For this review, take the finished solid that the model builds, in its own axes (mm). Face numbers are marked on the shaded views. A direction names the side the tool comes from. Coordinates: 2 decimals unless noted, no trailing zeros. Loops run counter-clockwise (first coordinate to the right, second up) from the corner with the lowest first, then second, coordinate; pieces in that order, holes last. Notation, with made-up numbers: M 19.25,-28.75 L 39.25,-28.75 A20 ccw 39.25,-23.75 Z; hole C 49,-29 d10. An arc over 180 degrees is marked long. Use one line per item in the form item = value.
```python
from build123d import *

# Parameters (mm, degrees)
SKETCH1_R                = 17.5
SKETCH1_R_2              = 1.45
FRONTPANEL_DEPTH         = 4
SKETCH1_3_R              = 34.7
SIDEWALLS_DEPTH          = 28.5
SKETCH2_R                = 19
MOTORSPACER_DEPTH        = 2
SKETCH1_5_R              = 1.45
MOTORMOUNTINGHOLES_DEPTH = 6
BOSS_EXTRUDE7_START      = -6.8
BOSS_EXTRUDE7_DEPTH      = 6.8
SKETCH3_5_R              = 2.2
CUT_EXTRUDE2_DEPTH       = 6
CUT_EXTRUDE8_DEPTH       = 65.705100263
SKETCH11_W               = 34
SKETCH11_H               = 28.5
BOSS_EXTRUDE8_DEPTH      = 10
SKETCH14_W               = 34
SKETCH14_H               = 31.5
BOSS_EXTRUDE9_DEPTH      = 1
CUT_EXTRUDE11_DEPTH      = 1
CUT_EXTRUDE11_DEPTH_BACK = 16
SKETCH19_R               = 10
SKETCH19_R_2             = 6
BOSS_EXTRUDE10_DEPTH     = 50
CUT_EXTRUDE12_REACH      = 227.811
CUT_EXTRUDE14_START      = -5
CUT_EXTRUDE14_DEPTH      = 215.755546028
CUT_EXTRUDE15_START      = -10
SKETCH19_6_R             = 6
CUT_EXTRUDE15_DEPTH      = 30


with BuildPart() as part:
    # Sketch1 → FrontPanel (new body)
    with BuildSketch(Plane.XY):
        with BuildLine():
            Line((-17, 34.543450899), (-17, 43.5))
            Line((-17, 43.5), (17, 43.5))
            Line((17, 43.5), (17, 34.543450899))
            ThreePointArc((17, 34.543450899), (0, -38.5), (-17, 34.543450899))
        make_face()
        Circle(SKETCH1_R, mode=Mode.SUBTRACT)
        with Locations((-7.749339505, 18.708560533)):
            Circle(SKETCH1_R_2, mode=Mode.SUBTRACT)
        with Locations((7.749339505, 18.708560533)):
            Circle(SKETCH1_R_2, mode=Mode.SUBTRACT)
        with Locations((18.708560533, 7.749339505)):
            Circle(SKETCH1_R_2, mode=Mode.SUBTRACT)
        with Locations((18.708560533, -7.749339505)):
            Circle(SKETCH1_R_2, mode=Mode.SUBTRACT)
        with Locations((7.749339505, -18.708560533)):
            Circle(SKETCH1_R_2, mode=Mode.SUBTRACT)
        with Locations((-7.749339505, -18.708560533)):
            Circle(SKETCH1_R_2, mode=Mode.SUBTRACT)
        with Locations((-18.708560533, -7.749339505)):
            Circle(SKETCH1_R_2, mode=Mode.SUBTRACT)
        with Locations((-18.708560533, 7.749339505)):
            Circle(SKETCH1_R_2, mode=Mode.SUBTRACT)
    extrude(amount=FRONTPANEL_DEPTH)

    # Sketch1<3> → SideWalls (add)
    with BuildSketch(Plane.XY):
        with BuildLine():
            Line((-17, 34.543450899), (-17, 43.5))
            Line((-17, 43.5), (17, 43.5))
            Line((17, 43.5), (17, 34.543450899))
            ThreePointArc((17, 34.543450899), (0, -38.5), (-17, 34.543450899))
        make_face()
        with Locations(Location((0, 0, 0), (0, 0, 180))):
            Circle(SKETCH1_3_R, mode=Mode.SUBTRACT)
    extrude(amount=SIDEWALLS_DEPTH)

    # Sketch2 → MotorSpacer (add)
    with BuildSketch(Plane.XY.offset(4)):
        with BuildLine():
            ThreePointArc((-5.4209, 21.321675431), (-9.088731519, 21.942138897), (-11.243546134, 18.909856434))
            ThreePointArc((-11.243546134, 18.909856434), (-15.556349186, 15.556349186), (-18.909856434, 11.243546134))
            ThreePointArc((-18.909856434, 11.243546134), (-21.942138897, 9.088731519), (-21.321675431, 5.4209))
            ThreePointArc((-21.321675431, 5.4209), (-22, 0), (-21.321675431, -5.4209))
            ThreePointArc((-21.321675431, -5.4209), (-21.942138897, -9.088731519), (-18.909856434, -11.243546134))
            ThreePointArc((-18.909856434, -11.243546134), (-15.556349186, -15.556349186), (-11.243546134, -18.909856434))
            ThreePointArc((-11.243546134, -18.909856434), (-9.088731519, -21.942138897), (-5.4209, -21.321675431))
            ThreePointArc((-5.4209, -21.321675431), (0, -22), (5.4209, -21.321675431))
            ThreePointArc((5.4209, -21.321675431), (9.088731519, -21.942138897), (11.243546134, -18.909856434))
            ThreePointArc((11.243546134, -18.909856434), (15.556349186, -15.556349186), (18.909856434, -11.243546134))
            ThreePointArc((18.909856434, -11.243546134), (21.942138897, -9.088731519), (21.321675431, -5.4209))
            ThreePointArc((21.321675431, -5.4209), (22, 0), (21.321675431, 5.4209))
            ThreePointArc((21.321675431, 5.4209), (21.942138897, 9.088731519), (18.909856434, 11.243546134))
            ThreePointArc((18.909856434, 11.243546134), (15.556349186, 15.556349186), (11.243546134, 18.909856434))
            ThreePointArc((11.243546134, 18.909856434), (9.088731519, 21.942138897), (5.4209, 21.321675431))
            ThreePointArc((5.4209, 21.321675431), (0, 22), (-5.4209, 21.321675431))
        make_face()
        with Locations(Location((0, 0, 0), (0, 0, 159.646622112))):
            Circle(SKETCH2_R, mode=Mode.SUBTRACT)
    extrude(amount=MOTORSPACER_DEPTH)

    # Sketch1<5> → MotorMountingHoles (cut)
    with BuildSketch(Plane.XY):
        with Locations(Location((-7.749339505, 18.708560533, 0), (0, 0, 263.105901259))):
            Circle(SKETCH1_5_R)
        with Locations(Location((7.749339505, 18.708560533, 0), (0, 0, 218.105901259))):
            Circle(SKETCH1_5_R)
        with Locations(Location((18.708560533, 7.749339505, 0), (0, 0, 173.105901259))):
            Circle(SKETCH1_5_R)
        with Locations(Location((18.708560533, -7.749339505, 0), (0, 0, 186.894098741))):
            Circle(SKETCH1_5_R)
        with Locations(Location((7.749339505, -18.708560533, 0), (0, 0, 141.894098741))):
            Circle(SKETCH1_5_R)
        with Locations(Location((-7.749339505, -18.708560533, 0), (0, 0, 96.894098741))):
            Circle(SKETCH1_5_R)
        with Locations(Location((-18.708560533, -7.749339505, 0), (0, 0, 51.894098741))):
            Circle(SKETCH1_5_R)
        with Locations(Location((-18.708560533, 7.749339505, 0), (0, 0, 308.105901259))):
            Circle(SKETCH1_5_R)
    extrude(amount=MOTORMOUNTINGHOLES_DEPTH, mode=Mode.SUBTRACT)

    # Sketch3 → Boss-Extrude7 (add)
    with BuildSketch(Plane.XY.offset(28.5).offset(BOSS_EXTRUDE7_START)):
        with BuildLine():
            Line((-21.775846711, 31.75), (-34.3, 31.75))
            Line((-34.3, 31.75), (-34.3, 17.485994396))
            ThreePointArc((-34.3, 17.485994396), (-28.930790001, 25.401956419), (-21.775846711, 31.75))
        make_face()
        with BuildLine():
            Line((34.3, 17.485994396), (34.3, 31.75))
            Line((34.3, 31.75), (21.775846711, 31.75))
            ThreePointArc((21.775846711, 31.75), (28.930790001, 25.401956419), (34.3, 17.485994396))
        make_face()
        with BuildLine():
            Line((-34.3, -17.485994396), (-34.3, -31.75))
            Line((-34.3, -31.75), (-21.775846711, -31.75))
            ThreePointArc((-21.775846711, -31.75), (-28.930790001, -25.401956419), (-34.3, -17.485994396))
        make_face()
        with BuildLine():
            Line((21.775846711, -31.75), (34.3, -31.75))
            Line((34.3, -31.75), (34.3, -17.485994396))
            ThreePointArc((34.3, -17.485994396), (28.930790001, -25.401956419), (21.775846711, -31.75))
        make_face()
    extrude(amount=BOSS_EXTRUDE7_DEPTH)

    # Sketch3<5> → Cut-Extrude2 (cut)
    with BuildSketch(Plane.XY.offset(28.5)):
        with Locations((-28.3, 25.75)):
            Circle(SKETCH3_5_R)
        with Locations(Location((28.3, 25.75, 0), (0, 0, 180))):
            Circle(SKETCH3_5_R)
        with Locations(Location((-28.3, -25.75, 0), (0, 0, 180))):
            Circle(SKETCH3_5_R)
        with Locations((28.3, -25.75)):
            Circle(SKETCH3_5_R)
    extrude(amount=-CUT_EXTRUDE2_DEPTH, mode=Mode.SUBTRACT)

    # Sketch7 → Cut-Extrude8 (cut, through all)
    with BuildSketch(Plane.XY.offset(28.5)):
        with BuildLine():
            Line((-4, 39.7), (4, 39.7))
            ThreePointArc((4, 39.7), (5.5, 38.2), (4, 36.7))
            Line((4, 36.7), (-4, 36.7))
            ThreePointArc((-4, 36.7), (-5.5, 38.2), (-4, 39.7))
        make_face()
    extrude(amount=-CUT_EXTRUDE8_DEPTH, mode=Mode.SUBTRACT)

    # Sketch14 → Boss-Extrude9 (add)
    with BuildSketch(Plane(origin=(0, 43.5, 0), x_dir=(1, 0, 0), z_dir=(0, 1, 0))):
        with Locations((0, -15.75)):
            Rectangle(SKETCH14_W, SKETCH14_H)
    extrude(amount=BOSS_EXTRUDE9_DEPTH)



with BuildPart() as body_2:
    # Sketch11 → Boss-Extrude8 (new body)
    with BuildSketch(Plane(origin=(0, 65, 0), x_dir=(1, 0, 0), z_dir=(0, 1, 0))):
        with Locations((0, -24.25)):
            Rectangle(SKETCH11_W, SKETCH11_H)
    extrude(amount=BOSS_EXTRUDE8_DEPTH)


with BuildPart() as part_1:
    add(part.part)

    add(body_2.part)  # loft5 joins it to this body
    # loft from a face of the part (loft5)
    loft([part_1.faces().sort_by_distance((0, 44.5, 15.75))[0], part_1.faces().sort_by_distance((0, 65, 24.25))[0]])

    # Sketch9 → Cut-Extrude11 (cut, two sides: drawn at the far end of the back side and taken through both)
    with BuildSketch(Plane(origin=(0, 34.7, 0), x_dir=(-1, 0, 0), z_dir=(0, -1, 0)).offset(-CUT_EXTRUDE11_DEPTH_BACK)):
        Polygon((-6.5, 0), (6.5, 0), (8, -3.2), (6.5, -3.2), (6.5, -8), (-6.5, -8), (-6.5, -3.2), (-8, -3.2), align=None)
    extrude(amount=CUT_EXTRUDE11_DEPTH + CUT_EXTRUDE11_DEPTH_BACK, mode=Mode.SUBTRACT)

    # Sketch19 → Boss-Extrude10 (add)
    # profile 1 of 3: a face of its own
    with BuildSketch(Plane(origin=(0, 0, 10), x_dir=(-1, 0, 0), z_dir=(0, 0, -1))):
        with BuildLine():
            Line((-17, 160), (-17, 75))
            Line((-17, 75), (-12, 75))
            Line((-12, 75), (-12, 127))
            ThreePointArc((-12, 127), (0, 139), (12, 127))
            Line((12, 127), (12, 75))
            Line((12, 75), (17, 75))
            Line((17, 75), (17, 160))
            ThreePointArc((17, 160), (15.720882745, 166.469454824), (12.076018151, 171.96535773))
            ThreePointArc((12.076018151, 171.96535773), (0, 177), (-12.076018151, 171.96535773))
            ThreePointArc((-12.076018151, 171.96535773), (-15.720882745, 166.469454824), (-17, 160))
        make_face()
        with Locations((0, 160)):
            Circle(SKETCH19_R, mode=Mode.SUBTRACT)
    # profile 2 of 3: a face of its own
    with BuildSketch(Plane(origin=(0, 0, 10), x_dir=(-1, 0, 0), z_dir=(0, 0, -1))):
        with BuildLine():
            Line((-12, 127), (-12, 75))
            Line((-12, 75), (12, 75))
            Line((12, 75), (12, 127))
            ThreePointArc((12, 127), (0, 139), (-12, 127))
        make_face()
    # profile 3 of 3: a face of its own
    with BuildSketch(Plane(origin=(0, 0, 10), x_dir=(-1, 0, 0), z_dir=(0, 0, -1))):
        with BuildLine():
            ThreePointArc((-10.332421948, 190.965011962), (-7.794094957, 181.152238037), (-12.076018151, 171.96535773))
            ThreePointArc((-12.076018151, 171.96535773), (0, 177), (12.076018151, 171.96535773))
            ThreePointArc((12.076018151, 171.96535773), (7.794094957, 181.152238037), (10.332421948, 190.965011962))
            ThreePointArc((10.332421948, 190.965011962), (0, 210.5), (-10.332421948, 190.965011962))
        make_face()
        with Locations((0, 198)):
            Circle(SKETCH19_R_2, mode=Mode.SUBTRACT)
    extrude(amount=-BOSS_EXTRUDE10_DEPTH)

    # Sketch21 → Cut-Extrude12 (cut, up to next)
    with BuildSketch(Plane(origin=(17, 0, 0), x_dir=(0, 0, -1), z_dir=(1, 0, 0)), mode=Mode.PRIVATE) as cut_extrude12_sk1:
        Polygon((-38.5, 75), (-60, 75), (-60, 137), align=None)
    cut_extrude12_tool1 = extrude(cut_extrude12_sk1.sketch, amount=-CUT_EXTRUDE12_REACH, mode=Mode.PRIVATE) & part_1.part
    add(cut_extrude12_tool1.solids().sort_by_distance((17, 95.666667, 52.833333))[0], mode=Mode.SUBTRACT)

    # Sketch19<5> → Cut-Extrude14 (cut, through all)
    with BuildSketch(Plane(origin=(0, 0, 10), x_dir=(-1, 0, 0), z_dir=(0, 0, -1)).offset(CUT_EXTRUDE14_START)):
        with BuildLine():
            Line((-12, 127), (-12, 75))
            Line((-12, 75), (12, 75))
            Line((12, 75), (12, 127))
            ThreePointArc((12, 127), (0, 139), (-12, 127))
        make_face()
        with BuildLine():
            Line((12, 75), (-12, 75))
            Line((-12, 75), (-12, 66.5))
            ThreePointArc((-12, 66.5), (-11.976447111, 65.748525049), (-11.9058809, 65))
            Line((-11.9058809, 65), (11.9058809, 65))
            ThreePointArc((11.9058809, 65), (11.976447111, 65.748525049), (12, 66.5))
            Line((12, 66.5), (12, 75))
        make_face()
        with BuildLine():
            Line((11.9058809, 65), (-11.9058809, 65))
            ThreePointArc((-11.9058809, 65), (0, 54.5), (11.9058809, 65))
        make_face()
    extrude(amount=-CUT_EXTRUDE14_DEPTH, mode=Mode.SUBTRACT)

    # Sketch19<6> → Cut-Extrude15 (cut)
    with BuildSketch(Plane(origin=(0, 0, 10), x_dir=(-1, 0, 0), z_dir=(0, 0, -1)).offset(CUT_EXTRUDE15_START)):
        with BuildLine():
            ThreePointArc((-10.332421948, 190.965011962), (-7.794094957, 181.152238037), (-12.076018151, 171.96535773))
            ThreePointArc((-12.076018151, 171.96535773), (0, 177), (12.076018151, 171.96535773))
            ThreePointArc((12.076018151, 171.96535773), (7.794094957, 181.152238037), (10.332421948, 190.965011962))
            ThreePointArc((10.332421948, 190.965011962), (0, 210.5), (-10.332421948, 190.965011962))
        make_face()
        with Locations((0, 198)):
            Circle(SKETCH19_6_R, mode=Mode.SUBTRACT)
    extrude(amount=-CUT_EXTRUDE15_DEPTH, mode=Mode.SUBTRACT)


solid = part_1.part
```
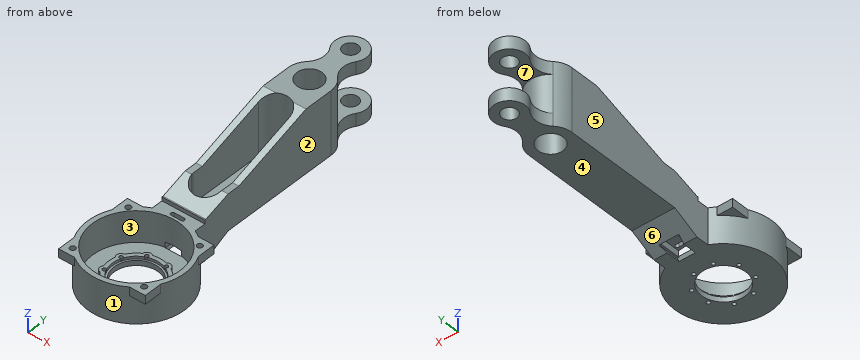
1. Consider section C-C on x = -28.3. Write out the cut boundary in (y, z), plus the area to 3 significant figures.
Computed values:
outline = M -31.75,21.7 L -26.1,21.7 L -26.1,0 L 26.1,0 L 26.1,21.7 L 31.75,21.7 L 31.75,28.5 L 27.95,28.5 L 27.95,22.5 L 23.55,22.5 L 23.55,28.5 L 20.08,28.5 L 20.08,4 L -20.08,4 L -20.08,28.5 L -23.55,28.5 L -23.55,22.5 L -27.95,22.5 L -27.95,28.5 L -31.75,28.5 Z
area = 528 mm2
2. For pin 1 Ø5 at (x, y) = (27.5, 24.5) entering from +Z; pin 2 Ø5 at (y, z) = (5.5, 31.5) entering from -X; pin 3 Ø23 at (x, y) = (3, -15.5) entering from +Z; pin 4 Ø3 at (x, y) = (-9.5, 64.5) entering from -Z, all flat-tipped, find the tip position at first contact; note any pin that passes through.
Computed values:
pin_1 = 28.5
pin_2 = through
pin_3 = 6
pin_4 = 9.02
3. Consider section A-A on y = 198. Write out the cut boundary in (x, z), plus the area to 3 significant figures.
Computed values:
outline = M -12.5,10 L -6,10 L -6,20 L -12.5,20 Z; M -12.5,50 L -6,50 L -6,60 L -12.5,60 Z; M 6,10 L 12.5,10 L 12.5,20 L 6,20 Z; M 6,50 L 12.5,50 L 12.5,60 L 6,60 Z
area = 260 mm2
4. Consider section B-B on y = 0. Write out the cut boundary in (x, z).
Computed values:
outline = M -38.5,0 L -17.5,0 L -17.5,4 L -19,4 L -19,6 L -22,6 L -22,4 L -34.7,4 L -34.7,28.5 L -38.5,28.5 Z; M 17.5,0 L 38.5,0 L 38.5,28.5 L 34.7,28.5 L 34.7,4 L 22,4 L 22,6 L 19,6 L 19,4 L 17.5,4 Z
5. Wall thickness on line 1 along Y through (x, z) = (0.5, 53.5); line 2 along Y through (x, z) = (0, 14.5); line 3 along Y through (x, z) = (-1.5, 56): over which ranges is each line inside the solid? List them lowest first. Write a range as from..to.
Computed values:
line_1 = 138.99..150.01, 169.99..192.02, 203.98..210.49
line_2 = -38.5..-34.7, 34.7..36.7, 39.7..150, 170..192, 204..210.5
line_3 = 138.91..150.11, 169.89..192.19, 203.81..210.41
6. Consider section D-D on x = 0.5. State how many separate pieces and enclosed holes the cut face has, plus the area to 3 significant figures.
Computed values:
separate_pieces = 7
enclosed_holes = 0
area = 2,450 mm2
7. Draft analysis for pull direction Z (two halves, no side actions). For the marked faces 5, 6 and 7, state which applies: +Z half, -Z half, draft (parallel to the pull), parting line (faces both ways), or undercut.
Computed values:
face_5 = draft
face_6 = -Z half
face_7 = undercut
8. Tool access review of the marked faces 1, 2, 3 and 4: name each direction out of +Z, -Z, +X, -X, +Y, -Y from which nothing blocks a thin tool from reaching the whole face with its end or side.
Computed values:
face_1 = -Z
face_2 = +Z, -Z, +X, +Y
face_3 = +Z
face_4 = -Z, +X, -X, +Y
